```python
from build123d import *

# Parameters (mm, degrees)
CROQUIS1_R                             = 5
SALIENTE_EXTRUIR1_DEPTH                = 43.5
CORTAR_EXTRUIR1_REACH                  = 46.071
CORTAR_EXTRUIR1_END_RADIUS             = 5
CROQUIS8_R                             = 1.5
CORTAR_EXTRUIR1_DIRECTION_2_REACH      = 46.071
CORTAR_EXTRUIR1_DIRECTION_2_END_RADIUS = 5
CORTAR_EXTRUIR2_REACH                  = 46.071
CROQUIS9_W                             = 2
CROQUIS9_H                             = 10
CORTAR_EXTRUIR2_DIRECTION_2_REACH      = 46.071


# Read off the part's stored shape, not the designer's step: Cortar-Revolución-Lámina1
with BuildPart() as part:
    # Croquis1 → Saliente-Extruir1 (new body)
    with BuildSketch(Plane(origin=(0, 0, 0), x_dir=(1, 0, 0), z_dir=(0, 1, 0))):
        with Locations(Location((0, 0, 0), (0, 0, 270))):
            Circle(CROQUIS1_R)
    extrude(amount=SALIENTE_EXTRUIR1_DEPTH)

    # Cortar-Revolución-Lámina1 outline → Cortar-Revolución-Lámina1 (revolve, cut)
    with BuildSketch(Plane.XY):
        Polygon((5, 43.5), (2.5, 43.5), (5, 33), align=None)
    revolve(axis=Axis((0, 0, 0), (0, 1, 0)), mode=Mode.SUBTRACT)

    # Cortar-Extruir1: up to this cylinder (the profile starts inside it)
    cortar_extruir1_end = Plane(origin=(0, 4.2, 0), z_dir=(0, -1, 0)) * Cylinder(CORTAR_EXTRUIR1_END_RADIUS, 103.142, mode=Mode.PRIVATE)
    # Croquis8 → Cortar-Extruir1 (cut, up to the surface)
    with BuildSketch(Plane(origin=(0, 0, 0), x_dir=(0, 0, -1), z_dir=(1, 0, 0)), mode=Mode.PRIVATE) as cortar_extruir1_sk1:
        with Locations(Location((0, 4.2, 0), (0, 0, 180))):
            Circle(CROQUIS8_R)
    cortar_extruir1_tool1 = extrude(cortar_extruir1_sk1.sketch, amount=-CORTAR_EXTRUIR1_REACH, mode=Mode.PRIVATE) & cortar_extruir1_end
    add(cortar_extruir1_tool1.solids().sort_by_distance((0, 4.2, 0))[0], mode=Mode.SUBTRACT)

    # Cortar-Extruir1 direction 2: up to this cylinder (the profile starts inside it)
    cortar_extruir1_direction_2_end = Plane(origin=(0, 4.2, 0), z_dir=(0, -1, 0)) * Cylinder(CORTAR_EXTRUIR1_DIRECTION_2_END_RADIUS, 103.142, mode=Mode.PRIVATE)
    # Croquis8 → Cortar-Extruir1 direction 2 (cut, up to the surface)
    with BuildSketch(Plane(origin=(0, 0, 0), x_dir=(0, 0, -1), z_dir=(1, 0, 0)), mode=Mode.PRIVATE) as cortar_extruir1_direction_2_sk1:
        with Locations(Location((0, 4.2, 0), (0, 0, 180))):
            Circle(CROQUIS8_R)
    cortar_extruir1_direction_2_tool1 = extrude(cortar_extruir1_direction_2_sk1.sketch, amount=CORTAR_EXTRUIR1_DIRECTION_2_REACH, mode=Mode.PRIVATE) & cortar_extruir1_direction_2_end
    add(cortar_extruir1_direction_2_tool1.solids().sort_by_distance((0, 4.2, 0))[0], mode=Mode.SUBTRACT)

    # Croquis9 → Cortar-Extruir2 (cut, up to next)
    with BuildSketch(Plane.XY, mode=Mode.PRIVATE) as cortar_extruir2_sk1:
        with Locations((0, 5)):
            Rectangle(CROQUIS9_W, CROQUIS9_H)
    cortar_extruir2_tool1 = extrude(cortar_extruir2_sk1.sketch, amount=-CORTAR_EXTRUIR2_REACH, mode=Mode.PRIVATE) & part.part
    add(cortar_extruir2_tool1.solids().sort_by_distance((0, 5, 0))[0], mode=Mode.SUBTRACT)

    # Croquis9 → Cortar-Extruir2 direction 2 (cut, up to next)
    with BuildSketch(Plane.XY, mode=Mode.PRIVATE) as cortar_extruir2_direction_2_sk1:
        with Locations((0, 5)):
            Rectangle(CROQUIS9_W, CROQUIS9_H)
    cortar_extruir2_direction_2_tool1 = extrude(cortar_extruir2_direction_2_sk1.sketch, amount=CORTAR_EXTRUIR2_DIRECTION_2_REACH, mode=Mode.PRIVATE) & part.part
    add(cortar_extruir2_direction_2_tool1.solids().sort_by_distance((0, 5, 0))[0], mode=Mode.SUBTRACT)


solid = part.part
```
Check sheet for the modelled part. Datum: model origin and axes. Units: mm. A direction names the side the tool comes from. Coordinates: 2 decimals unless noted, no trailing zeros. Order: outer loops, then holes, each group sorted by start corner. A loop starts at its lowest first (then second) coordinate and runs counter-clockwise, first axis right, second up. Notation, with made-up numbers: M 37,-33.5 L 61,-33.5 A23 ccw 61,-9.5 Z; hole C -35,70.25 d3. An arc over 180 degrees is marked long. Write each question's results on one line, items separated by ' | '. Start each with the question number.
1. Cross-section at A-A on z = 0. Record the cut outline in (x, y).
2. Go/stop test with flat-tipped pins: P1, Ø2, axis at y = 35, z = 3, coming from the -X side; P2, Ø6, axis at x = 1.5, y = 34.5, coming from the +Z side. Record where each tip stops, or that it passes through.
3. Access from +Z, -Z, +X, -X, +Y, -Y to the whole of each face (thin tool, end or side, straight path). Record for faces 1 (the face through (-3, 0, 0)), 2 (the face through (-1, 6, 0)).
4. Cross-section at C-C on x = 0. Record the cut outline in (y, z), and give its area (3 significant figures).
5. Cross-section at B-B on y = 4.2. Record the cut outline in (x, z), and give its area (3 significant figures).
6. Material ranges on probe 1 along Y at (x, z) = (-2.4, 0); probe 2 along X at (y, z) = (2, 2.5); probe 3 along Y at (x, z) = (0.5, -1), recorded low to high.
7. Cross-section at D-D on y = 19. Record the cut outline in (x, z).
8. Mould release check, pull along Z, two halves, no side actions. Record for faces 3 (the face through (0, 10, 0)), 4 (the face through (-1.915, 16.269, 4.619)), 5 (the face through (-2.975, 2.935, 0.806)): +Z half, -Z half, draft (parallel to the pull), parting line (faces both ways), or undercut.
Checks:
1) outline: M -5,0 L -1,0 L -1,2.7 L -5,2.7 Z; M -5,5.7 L -1,5.7 L -1,10 L 1,10 L 1,5.7 L 5,5.7 L 5,33 L 2.5,43.5 L -2.5,43.5 L -5,33 Z; M 1,0 L 5,0 L 5,2.7 L 1,2.7 Z
2) P1: stops at x = -4.12 | P2: stops at z = 5
3) face 1: +Z, -Z, +X, -X, -Y | face 2: +Z, -Z, -Y
4) outline: M 10,-5 L 33,-5 L 43.5,-2.5 L 43.5,2.5 L 33,5 L 10,5 Z | area: 309 mm²
5) outline: M -4.77,-1.5 A5 ccw -1,-4.9 L -1,-1.5 Z; M -4.77,1.5 L -1,1.5 L -1,4.9 A5 ccw Z; M 1,-4.9 A5 ccw 4.77,-1.5 L 1,-1.5 Z; M 1,1.5 L 4.77,1.5 A5 ccw 1,4.9 Z | area: 35.1 mm²
6) probe 1: y = 0 to 2.7, 5.7 to 43.5 | probe 2: x = -4.33 to -1, 1 to 4.33 | probe 3: y = 10 to 43.5
7) outline: C 0,0 d10
8) face 3: draft | face 4: parting line | face 5: undercut
